Autodesk Inventor part; units mm, degrees
ref_plane "YZ Plane" through (0, 0, 0) normal (1, 0, 0) x (0, 1, 0)
ref_plane "XZ Plane" through (0, 0, 0) normal (0, 1, 0) x (-1, 0, 0)
ref_plane "XY Plane" through (0, 0, 0) normal (0, 0, 1) x (1, 0, 0)
sketch "Sketch1" plane through (0, 0, 0) normal (0, 0, 1) x (1, 0, 0)
  circle A0 centre (0, 0) radius 4
  dimension "d0" = 8
extrude "Extrusion1" add sketch "Sketch1" along normal blind 10.5
sketch "Sketch2" plane through (0, 0, 0) normal (1, 0, 0) x (0, 1, 0)
  line L0 (4.5, 9) -> (3.5, 9)
  line L1 (3.5, 9) -> (3.5, 8.06)
  line L2 (3.5, 8.06) -> (4.5, 8.06)
  line L3 (4.5, 8.06) -> (4.5, 9)
  line L4 (4, 0) -> (4, 10.5)
  line L5 (4, 10.5) -> (-4, 10.5)
  line L6 (0, -2.2) -> (0, 13.2)
  line L7 (2.4774, 8) -> (9.7598, 8)
  point P0 (0, 0)
  dimension "d3" = 0.5
  dimension "d4" = 1
  dimension "d5" = 0.94
  dimension "d6" = 1.5
revolve "Revolution1" cut sketch "Sketch2" angle 360 about axis through (0, 0, -10) along (0, 0, 1)
equation "\"d4\" = 2 * d3"
properties part number "AxeJambe" material "Stainless Steel"
Input: part model. Units: mm. Frame: model coordinates. Give positions to 0.01 mm unless a question says otherwise; leave off trailing zeros. Order: outer loops, then holes, each group sorted by start corner. A loop starts at its lowest first (then second) coordinate and runs counter-clockwise, first axis right, second up.
1. Section A-A on y = 1.25. Return the cut outline in (x, z), and give its area (3 significant figures).
Derived:
outline: (-3.8, 0) - (3.8, 0) - (3.8, 8.06) - (3.27, 8.06) - (3.27, 9) - (3.8, 9) - (3.8, 10.5) - (-3.8, 10.5) - (-3.8, 9) - (-3.27, 9) - (-3.27, 8.06) - (-3.8, 8.06) - close
area: 78.8 mm2
2. Section C-C on z = 2.75. Return the cut outline in (x, y).
Derived:
outline: circle Ø8 at (0, 0)
3. Section B-B on x = 2.5. Return the cut outline in (y, z), and give its area (3 significant figures).
Derived:
outline: (-3.12, 0) - (3.12, 0) - (3.12, 8.06) - (2.45, 8.06) - (2.45, 9) - (3.12, 9) - (3.12, 10.5) - (-3.12, 10.5) - (-3.12, 9) - (-2.45, 9) - (-2.45, 8.06) - (-3.12, 8.06) - close
area: 64.3 mm2
4. Mould query, pull axis Z, two halves, no side actions, for faces 1 (the cylindrical face through (-1.341, 3.233, 8.523)), 2 (the flat face through (0, 0, 10.5)), 3 (the cylindrical face through (-0.867, 3.905, 3.974)). Classes: released by +Z, released by -Z, zero draft, split by the parting line, or undercut.
Derived:
face 1: undercut
face 2: released by +Z
face 3: zero draft
5. Material intervals for L1, parallel to Z at x = 1.75, y = -3.5; L2, parallel to Y at x = -3.5, z = 3; L3, parallel to X at y = 2.25, z = 5.25, sorted ascending.
Derived:
L1: z = 0 to 8.06, 9 to 10.5
L2: y = -1.94 to 1.94
L3: x = -3.31 to 3.31
